Geometry check sheet. Reference: the model listing, model coordinates, mm. Face numbers are marked on the shaded views. A direction names the side the tool comes from. Coordinates: 2 decimals unless noted, no trailing zeros. Loops run counter-clockwise (first coordinate to the right, second up) from the corner with the lowest first, then second, coordinate; pieces in that order, holes last. Notation, with made-up numbers: M 36.5,-26.75 L 95.5,-26.75 A18 cw 95.5,0.25 Z; hole C 54,87 d4. An arc over 180 degrees is marked long. One line per question, with ' | ' between items. Start each with the question number.
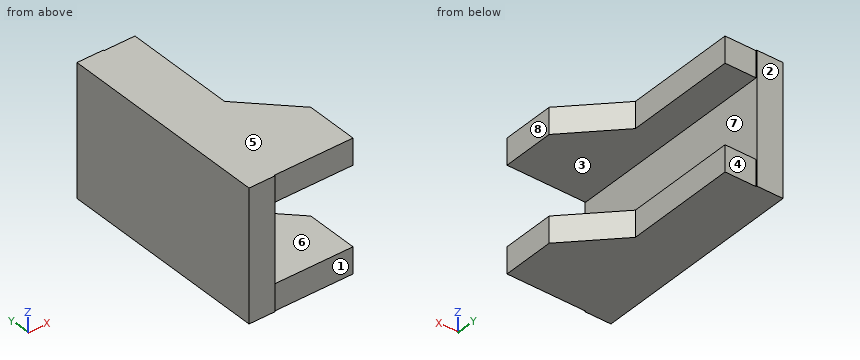
from build123d import *

# Parameters (mm, degrees)
F0_W     = 77.7875
F0_H     = 47.625
F1_DEPTH = 9.525
F2_R     = 12.6438150781
F3_DEPTH = 97
F5_DEPTH = 9.525


# Not quite as in the source:
# - an extrude ends at something that could not be found from the text; its depth is read off the source's solid


with BuildPart() as f1:
    # F0 (on Right) → F1 (new body)
    with BuildSketch(Plane.YZ):
        Rectangle(F0_W, F0_H)
    extrude(amount=F1_DEPTH)

    # F2 (on Right) → F3 (cut, through all)
    with BuildSketch(Plane.YZ):
        Circle(F2_R)
    extrude(amount=-F3_DEPTH, mode=Mode.SUBTRACT)

    # F4 (on face) → F5 (join)
    with BuildSketch(Plane.XY.offset(23.8125)):
        Polygon((0, 38.5659709573), (0, -38.5659709573), (38.1, -38.5659709573), (38.1, -19.5159709573), (20.8316552401, -1.9598177195), (20.8316552401, 38.5659709573), align=None)
    extrude(amount=-F5_DEPTH)

    # F6: F1 across plane


with BuildPart() as f1_1:
    add(f1.part)
    add(f1.part.mirror(Plane.XY))


solid = f1_1.part
1. Sectioned sample at D-D (x = 36). Record the cut outline in (y, z), and give its area (3 significant figures).
2. Draft check along Z on the marked faces 5, 6, 7 and 8. Enter one of: +Z half, -Z half, draft (parallel to the pull), parting line (faces both ways), or undercut.
3. Depth check by flat-ended pin: pin 1 Ø1 at (y, z) = (20, 12.5) entering from +X (3 decimals); pin 2 Ø5 at (y, z) = (11.5, 21.5) entering from +X; pin 3 Ø5 at (x, z) = (26, -20.5) entering from -Y. Enter the tip coordinate at first touch or a pass-through.
4. Sectioned sample at A-A (x = 29.5). Record the cut outline in (y, z).
5. Sectioned sample at C-C (y = 24). Record the cut outline in (x, z) (1 decimal), and give its area (3 significant figures).
6. Sectioned sample at B-B (z = -17). Record the cut outline in (x, y) (3 decimals).
7. Tool access check on the marked faces 1, 2, 3 and 4. Record the directions out of +Z, -Z, +X, -X, +Y, -Y that give a thin tool (end or side, any length) a straight path to the whole face; none if there is none.
8. Thickness scan on line 1 (Z direction, x = 34, y = -33.5); line 2 (X direction, y = -15, z = 1) (3 decimals); line 3 (X direction, y = 1.5, z = 20). Record the ranges inside material, lowest first.
Result:
1) outline: M -38.57,-23.81 L -17.38,-23.81 L -17.38,-14.29 L -38.57,-14.29 Z; M -38.57,14.29 L -17.38,14.29 L -17.38,23.81 L -38.57,23.81 Z | area: 404 mm2
2) face 5: +Z half | face 6: undercut | face 7: undercut | face 8: draft
3) pin 1: stops at x = 9.525 | pin 2: stops at x = 20.83 | pin 3: stops at y = -38.57
4) outline: M -38.57,-23.81 L -10.77,-23.81 L -10.77,-14.29 L -38.57,-14.29 Z; M -38.57,14.29 L -10.77,14.29 L -10.77,23.81 L -38.57,23.81 Z
5) outline: M 0,-23.8 L 20.8,-23.8 L 20.8,-14.3 L 9.5,-14.3 L 9.5,14.3 L 20.8,14.3 L 20.8,23.8 L 0,23.8 Z | area: 669 mm2
6) outline: M 0,-38.894 L 9.525,-38.894 L 9.525,-38.566 L 38.1,-38.566 L 38.1,-19.516 L 20.832,-1.96 L 20.832,38.566 L 9.525,38.566 L 9.525,38.894 L 0,38.894 Z
7) face 1: +Z, -Z, +X, -Y | face 2: +Z, -Z, +X, -X, +Y | face 3: +X, +Y, -Y | face 4: +Z, -Z, +X, +Y
8) line 1: z = -23.81 to -14.29, 14.29 to 23.81 | line 2: x = 0 to 9.525 | line 3: x = 0 to 20.83
